Check sheet for the modelled part. Datum: model origin and axes. Units: mm. A direction names the side the tool comes from. Round coordinates to 2 decimals unless told otherwise and drop trailing zeros. Order: outer loops, then holes, each group sorted by start corner. A loop starts at its lowest first (then second) coordinate and runs counter-clockwise, first axis right, second up. Notation, with made-up numbers: (42.5, 3) -> (61.5, 3) arc R27 ccw to (61.5, 33) -> close; hole circle Ø11 at (55.5, -33.75). An arc over 180 degrees is marked (long way). Use CSV: the item, a comma, the result in double quotes.
Autodesk Inventor part; units mm, degrees
ref_plane "YZ Plane" through (0, 0, 0) normal (1, 0, 0) x (0, 1, 0)
ref_plane "XZ Plane" through (0, 0, 0) normal (0, 1, 0) x (-1, 0, 0)
ref_plane "XY Plane" through (0, 0, 0) normal (0, 0, 1) x (1, 0, 0)
sketch "Sketch1" plane through (0, 0, 0) normal (0, 1, 0) x (-1, 0, 0)
  line L0 (33.75, 44.75) -> (-33.75, 44.75)
  line L1 (-33.75, 44.75) -> (-33.75, -44.75)
  line L2 (-33.75, -44.75) -> (33.75, -44.75)
  line L3 (33.75, -44.75) -> (33.75, 44.75)
  line L4 (21.75, -36.75) -> (-21.75, -36.75)
  line L5 (21.75, 36.75) -> (-21.75, 36.75)
  line L6 (21.75, 36.75) -> (21.75, -36.75)
  line L7 (-21.75, 36.75) -> (-21.75, -36.75)
  line L8 (33.75, -41.75) -> (-33.75, -41.75)
  line L9 (33.75, 41.75) -> (-33.75, 41.75)
  point P0 (0, 0)
  point P1 (-33.75, 0)
  dimension "d0" = 83.5
  dimension "d1" = 3
  dimension "d2" = 3
  dimension "d4" = 5
  dimension "d5" = 5
  dimension "d6" = 12
  dimension "d7" = 12
  dimension "d8" = 67.5
  dimension "d9" = 33.75
  dimension "d10" = 41.75
extrude "Extrusion1" add sketch "Sketch1" along normal blind 2 contours L3 L8 L1 L9
extrude "Extrusion2" add sketch "Sketch1" along normal blind 32 and the other way blind 4 contours L3 L9 L1 L0 | L3 L2 L1 L8
sketch "Sketch2" plane through (0, 32, 0) normal (0, 1, 0) x (1, 0, 0)
  line L0 (33.75, -44.75) -> (33.75, -41.75)
  line L1 (33.75, -41.75) -> (-33.75, -41.75)
  line L2 (-33.75, -41.75) -> (-33.75, -44.75)
  line L3 (-33.75, -44.75) -> (33.75, -44.75)
  line L4 (-33.75, 44.75) -> (-33.75, 41.75)
  line L5 (-33.75, 41.75) -> (33.75, 41.75)
  line L6 (33.75, 41.75) -> (33.75, 44.75)
  line L7 (33.75, 44.75) -> (-33.75, 44.75)
  line L8 (-33.75, 41.75) -> (-33.75, -41.75)
  line L9 (33.75, -41.75) -> (33.75, 41.75)
  line L10 (-33.75, 34.75) -> (24.75, 34.75)
  line L11 (-33.75, -34.75) -> (24.75, -34.75)
  line L12 (24.75, -34.75) -> (24.75, 0)
  line L13 (24.75, 0) -> (24.75, 34.75)
  line L14 (-33.75, -34.75) -> (-65.75, 0)
  line L15 (-65.75, 0) -> (-33.75, 34.75)
  line L16 (33.75, 44.75) -> (33.75, 0)
  line L17 (33.75, -41.75) -> (33.75, -44.75)
  line L18 (33.75, 0) -> (33.75, -44.75)
  line L19 (-33.75, -44.75) -> (-76.75, 0)
  line L20 (-33.75, 44.75) -> (-33.75, 41.75)
  line L21 (-76.75, 0) -> (-33.75, 44.75)
  point P0 (0, 0)
  dimension "d18" = 7
  dimension "d19" = 7
  dimension "d20" = 110.5
  dimension "d21" = 90.5
  dimension "d42" = 9
extrude "Extrusion3" add sketch "Sketch2" along normal blind 3 contours L3 L2 L1 L0 | L1 L8 L11 L12 L13 L10 L5 L9 | L19 L21 L4 L8 L15 L14 L2 | L5 L4 L7 L6
sketch "Sketch3" plane through (0, 35, 0) normal (0, 1, 0) x (1, 0, 0)
  circle A0 centre (29.25, 0) radius 4.5
  circle A1 centre (-70.45, 0) radius 4.5
  circle A2 centre (-70.45, 0) radius 2.35
  circle A3 centre (29.25, 0) radius 2.35
  line L0 (33.75, -44.75) -> (33.75, 44.75)
  point P0 (0, 0)
  dimension "d24" = 9
  dimension "d27" = 4.7
  dimension "d43" = 99.7
  dimension "d44" = 4.5
extrude "Extrusion4" add sketch "Sketch3" along normal blind 2.15
extrude "Extrusion5" cut sketch "Sketch3" against normal blind 3 contours A2 | A3
sketch "Sketch4" plane through (0, 2, 0) normal (0, 1, 0) x (1, 0, 0)
  circle A0 centre (-25.8, -33) radius 2.35
  circle A1 centre (-25.8, 33) radius 2.35
  circle A2 centre (25.8, -33) radius 2.35
  circle A3 centre (25.8, 33) radius 2.35
  line L0 (-33.75, 41.75) -> (-33.75, -41.75)
  line L1 (-33.75, -41.75) -> (33.75, -41.75)
  line L2 (33.75, -41.75) -> (33.75, 41.75)
  line L3 (33.75, 41.75) -> (-33.75, 41.75)
  point P0 (0, 0)
  dimension "d35" = 4.7
  dimension "d36" = 7.95
  dimension "d37" = 8.75
  dimension "d38" = 7.95
  dimension "d39" = 8.75
extrude "Extrusion6" cut sketch "Sketch4" against normal blind 3 contours A0 | A1 | A2 | A3
fillet "Fillet1" radius 4 9 edges at (-33.75, 33.5, 34.75) (-65.75, 33.5, 0) (-33.75, 33.5, -34.75) (24.75, 33.5, 34.75) (24.75, 33.5, -34.75) (21.75, 1, 36.75) (21.75, 1, -36.75) (-21.75, 1, 36.75) (-21.75, 1, -36.75)
equation "\"d2\" = d1"
equation "\"d5\" = d4"
equation "\"d7\" = d6"
equation "\"d19\" = d18"
equation "\"d44\" = 0.5 * d24"
equation "\"d38\" = d36"
equation "\"d39\" = d37"
properties part number "CO-1-01-fuseMount"
Q1. Sectioned sample at C-C, the plane x = -70.45. Enter the section's corners in (y, z), then the cut area to 3 significant figures.
Result sheet:
outline,"(32, -6.56) -> (35, -6.56) -> (35, -4.5) -> (37.15, -4.5) -> (37.15, -2.35) -> (32, -2.35) -> close; (32, 2.35) -> (37.15, 2.35) -> (37.15, 4.5) -> (35, 4.5) -> (35, 6.56) -> (32, 6.56) -> close"
area,"34.5 mm^2"
Q2. Go/stop test with flat-tipped pins: pin 1 (1.5 mm diameter, centred on x = -42, z = 30.5, fed in from +Y); pin 2 (6 mm diameter, centred on x = 22, z = 22.5, fed in from -Y); pin 3 (3 mm diameter, centred on x = -52.5, y = 29, fed in from -Z); pin 4 (12 mm diameter, centred on y = 26.5, z = 6, fed in from -X). Record where each tip stops, or that it passes through.
Result sheet:
pin 1,"stops at y = 35"
pin 2,"stops at y = 0"
pin 3,"passes through"
pin 4,"stops at x = -73.29"
Q3. Sectioned sample at D-D, the plane z = -21.5. Enter the section's corners in (x, y).
Result sheet:
outline,"(-56.09, 32) -> (-45.95, 32) -> (-45.95, 35) -> (-56.09, 35) -> close; (-33.75, 0) -> (-21.75, 0) -> (-21.75, 2) -> (-33.75, 2) -> close; (21.75, 0) -> (33.75, 0) -> (33.75, 2) -> (21.75, 2) -> close; (24.75, 32) -> (33.75, 32) -> (33.75, 35) -> (24.75, 35) -> close"
Q4. Sectioned sample at A-A, the plane y = 7. Enter the section's corners in (x, z).
Result sheet:
outline,"(-33.75, -44.75) -> (33.75, -44.75) -> (33.75, -41.75) -> (-33.75, -41.75) -> close; (-33.75, 41.75) -> (33.75, 41.75) -> (33.75, 44.75) -> (-33.75, 44.75) -> close"
Q5. Access from +Z, -Z, +X, -X, +Y, -Y to the whole of each face (thin tool, end or side, straight path). Record for faces 1 (the face through (-33.75, 1, 0)), 2 (the face through (-49.295, 33.479, -17.869)), 3 (the face through (-26.11, 1.01, -35.33)), 4 (the face through (-6, 33, -34.75)), 5 (the face through (-22, 2, 1)).
Result sheet:
face 1,"+Z, -Z, -X, -Y"
face 2,"+Y, -Y"
face 3,"-Y"
face 4,"+Y"
face 5,"+X, -X"
Q6. Sectioned sample at B-B, the plane x = -25.8. Enter the section's corners in (y, z).
Result sheet:
outline,"(-4, -44.75) -> (35, -44.75) -> (35, -34.75) -> (32, -34.75) -> (32, -41.75) -> (2, -41.75) -> (2, -35.35) -> (0, -35.35) -> (0, -41.75) -> (-4, -41.75) -> close; (-4, 41.75) -> (0, 41.75) -> (0, 35.35) -> (2, 35.35) -> (2, 41.75) -> (32, 41.75) -> (32, 34.75) -> (35, 34.75) -> (35, 44.75) -> (-4, 44.75) -> close; (0, -30.65) -> (2, -30.65) -> (2, 30.65) -> (0, 30.65) -> close"
Q7. Scan lines: L1, parallel to X at y = 35.8, z = 0; L2, parallel to Z at x = 25.8, y = 1.45; L3, parallel to X at y = 34.35, z = 0. Record each from-to range of solid material in increasing order.
Result sheet:
L1,"x = -74.95 to -72.8, -68.1 to -65.95, 24.75 to 26.9, 31.6 to 33.75"
L2,"z = -44.75 to -35.35, -30.65 to 30.65, 35.35 to 44.75"
L3,"x = -76.75 to -72.8, -68.1 to -64.31, 24.75 to 26.9, 31.6 to 33.75"
Q8. Mould release check, pull along Y, two halves, no side actions. Record for faces 6 (the face through (-68.5, 37.15, 1.9)), 7 (the face through (24.75, 33, 0)), 8 (the face through (0, 17, 41.75)), 9 (the face through (0, -4, -43)): pulls with the +Y half, pulls with the -Y half, needs draft (parallel to the pull), parting line crosses it, or undercut.
Result sheet:
face 6,"pulls with the +Y half"
face 7,"needs draft"
face 8,"undercut"
face 9,"pulls with the -Y half"
